Geometry: final body of the model. Coordinates: model frame, mm. Give positions to 0.01 mm unless a question says otherwise; leave off trailing zeros. Write each loop counter-clockwise with the first axis right and the second up, starting at its lowest first coordinate (ties: lowest second). Pieces come first, ordered by that corner, then holes. Notation, with made-up numbers: (-38.5, 87) -> (7.5, 87) arc R14 cw to (7.5, 113) -> close; hole circle Ø10 at (2, -5.5). An arc over 180 degrees is marked (long way). Answer as a JSON object with one key per item and string values.
from build123d import *

# Parameters (mm, degrees)
F0_W     = 14.9271550402
F0_H     = 6
F0_H_2   = 10
F1_DEPTH = 1
F2_R     = 0.25
F3_DEPTH = 1
F0_W_2   = 6
F0_H_3   = 12
F4_DEPTH = 1
F5_R     = 0.5


# Not quite as in the source:
# - a feature names something its author has since deleted; it is built from what else it names


with BuildPart() as f1:
    # F0 (on Top) → F1 (new body)
    with BuildSketch(Plane.XY):
        with Locations((-0.0364224799, 10.5)):
            Rectangle(F0_W, F0_H)
        Polygon((7.4271550402, 7.5), (-7.5, 7.5), (-7.5, -7.5), (7.4271550402, -7.5), (7.5, -7.5), (7.5, -6.1350027099), (7.5, 5.8649972901), (7.5, 7.5), align=None)
        with BuildLine():
            ThreePointArc((-5, 0), (-4.267766953, 1.767766953), (-2.5, 2.5))
            Line((-2.5, 2.5), (2.5, 2.5))
            ThreePointArc((2.5, 2.5), (4.267766953, 1.767766953), (5, 0))
            ThreePointArc((5, 0), (4.267766953, -1.767766953), (2.5, -2.5))
            Line((2.5, -2.5), (-2.5, -2.5))
            ThreePointArc((-2.5, -2.5), (-4.267766953, -1.767766953), (-5, 0))
        make_face(mode=Mode.SUBTRACT)
        with Locations((-0.0364224799, -12.5)):
            Rectangle(F0_W, F0_H_2)
    extrude(amount=F1_DEPTH)

    # F2
    f2_edges = [f1.edges().sort_by_distance(p)[0] for p in [
        (-0.036422, 13.5, 0),
        (-7.5, -2, 0),
        (-0.036422, -17.5, 0),
        (7.427155, -12.5, 0),
        (7.463578, -7.5, 0),
        (7.5, 0, 0),
        (7.463578, 7.5, 0),
        (7.427155, 10.5, 0),
        (-5, 0, 0),
        (0, 2.5, 0),
        (5, 0, 0),
        (0, -2.5, 0),
    ]]
    fillet(f2_edges, radius=F2_R)

    # F0 (on Top) → F3 (cut)
    with BuildSketch(Plane.XY):
        with BuildLine():
            Line((2.5, 2.5), (-2.5, 2.5))
            ThreePointArc((-2.5, 2.5), (-4.267766953, 1.767766953), (-5, 0))
            ThreePointArc((-5, 0), (-4.267766953, -1.767766953), (-2.5, -2.5))
            Line((-2.5, -2.5), (2.5, -2.5))
            ThreePointArc((2.5, -2.5), (4.267766953, -1.767766953), (5, 0))
            ThreePointArc((5, 0), (4.267766953, 1.767766953), (2.5, 2.5))
        make_face()
    extrude(amount=F3_DEPTH, mode=Mode.SUBTRACT)

    # F0 (on Top) → F4 (join)
    with BuildSketch(Plane.XY):
        with Locations((10.5, -0.1350027099)):
            Rectangle(F0_W_2, F0_H_3)
    extrude(amount=F4_DEPTH)

    # F5
    f5_edges = [f1.edges().sort_by_distance(p)[0] for p in [
        (-0.036422, 13.5, 1),
        (-7.5, -2, 1),
        (-0.036422, -17.5, 1),
        (7.427155, -12.5, 1),
        (7.463578, -7.5, 1),
        (7.5, -6.817501, 1),
        (10.5, -6.135003, 1),
        (13.5, -0.135003, 1),
        (10.5, 5.864997, 1),
        (7.5, 6.682499, 1),
        (7.463578, 7.5, 1),
        (7.427155, 10.5, 1),
        (-5, 0, 1),
        (0, 2.5, 1),
        (5, 0, 1),
        (0, -2.5, 1),
    ]]
    fillet(f5_edges, radius=F5_R)


solid = f1.part
Q1. Cut plane D-D (x = 9). Return the cut outline in (y, z) (3 decimals), and give its area (3 significant figures).
Values:
{"outline": "(-6.135, 0) -> (5.865, 0) -> (5.865, 0.5) arc R0.5 ccw to (5.365, 1) -> (-5.635, 1) arc R0.5 ccw to (-6.135, 0.5) -> close", "area": "11.9 mm²"}
Q2. Cut plane B-B (y = 10). Return the cut outline in (x, z).
Values:
{"outline": "(-7.5, 0.25) arc R0.25 ccw to (-7.25, 0) -> (7.18, 0) arc R0.25 ccw to (7.43, 0.25) -> (7.43, 0.5) arc R0.5 ccw to (6.93, 1) -> (-7, 1) arc R0.5 ccw to (-7.5, 0.5) -> close"}
Q3. Material intervals for L1, parallel to X at y = -7, z = 0.3; L2, parallel to X at y = -12.5, z = 0.3; L3, parallel to Y at x = 10, z = 0.3 (3 decimals), sorted ascending. Write a range as from..to.
Values:
{"L1": "-7.5..7.5", "L2": "-7.5..7.43", "L3": "-6.135..5.865"}
Q4. First-contact query: P1, Ø0.6, axis at x = 11.5, z = 0, coming from the -Y side (3 decimals). Flat tip, straight axial feed; report the tip coordinate or a pass-through.
Values:
{"P1": "y = -6.135"}
Q5. Cut plane C-C (z = 0.75). Return the cut outline in (x, y), and give its area (3 significant figures).
Values:
{"outline": "(-7.43, -17.43) -> (7.36, -17.43) -> (7.36, -7.43) -> (7.43, -7.43) -> (7.43, -6.07) -> (13.43, -6.07) -> (13.43, 5.8) -> (7.43, 5.8) -> (7.43, 7.43) -> (7.36, 7.43) -> (7.36, 13.43) -> (-7.43, 13.43) -> close; hole (-2.5, -2.57) -> (2.5, -2.57) arc R2.57 ccw to (2.5, 2.57) -> (-2.5, 2.57) arc R2.57 ccw to start", "area": "483 mm²"}
Q6. Cut plane A-A (x = 2). Return the cut outline in (y, z), and give its area (3 significant figures).
Values:
{"outline": "(-17.5, 0.25) arc R0.25 ccw to (-17.25, 0) -> (-2.75, 0) arc R0.25 ccw to (-2.5, 0.25) -> (-2.5, 0.5) arc R0.5 ccw to (-3, 1) -> (-17, 1) arc R0.5 ccw to (-17.5, 0.5) -> close; (2.5, 0.25) arc R0.25 ccw to (2.75, 0) -> (13.25, 0) arc R0.25 ccw to (13.5, 0.25) -> (13.5, 0.5) arc R0.5 ccw to (13, 1) -> (3, 1) arc R0.5 ccw to (2.5, 0.5) -> close", "area": "25.7 mm²"}
